Verification items for this drawing (mm, ordinates from the low corner). Coordinates: 2 decimals unless noted, no trailing zeros. Write each loop counter-clockwise with the first axis right and the second up, starting at its lowest first coordinate (ties: lowest second). Pieces come first, ordered by that corner, then holes.
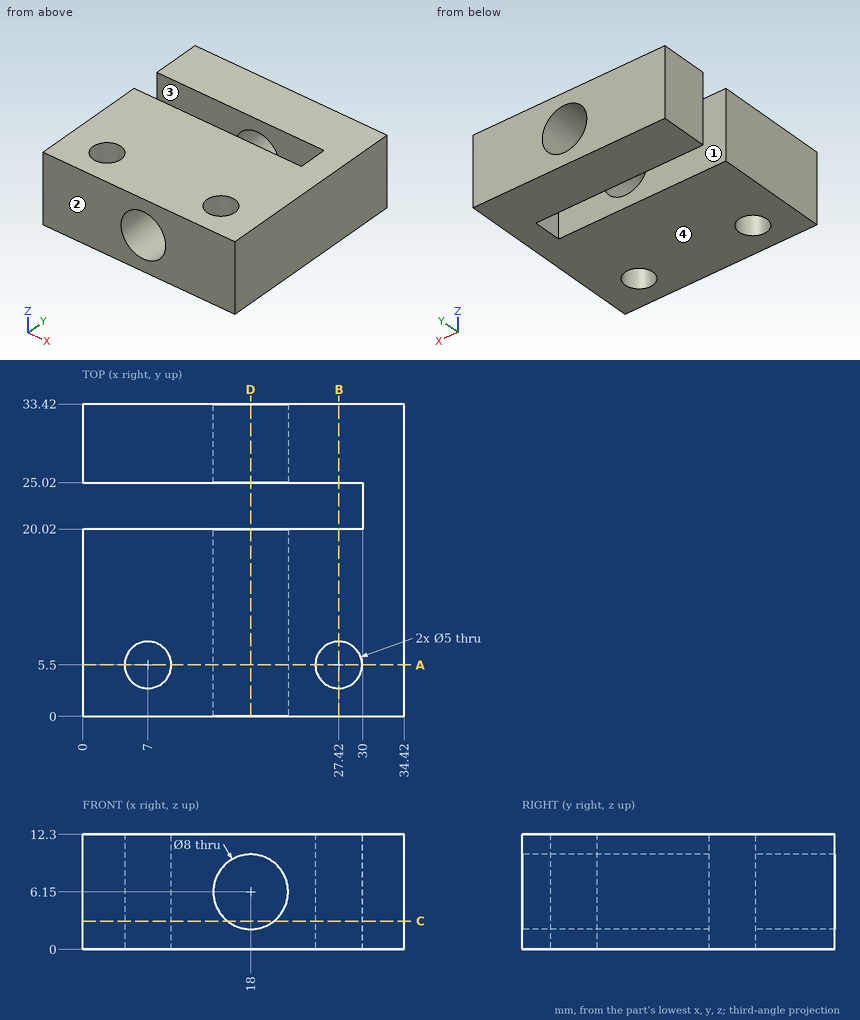
1. Sectioned sample at D-D, the plane x = 18. Record the boundary of the cut face in (y, z).
Computed values:
outline: (0, 0) - (20.02, 0) - (20.02, 2.15) - (0, 2.15) - close; (0, 10.15) - (20.02, 10.15) - (20.02, 12.3) - (0, 12.3) - close; (25.02, 0) - (33.42, 0) - (33.42, 2.15) - (25.02, 2.15) - close; (25.02, 10.15) - (33.42, 10.15) - (33.42, 12.3) - (25.02, 12.3) - close
2. Thickness scan on line 1 along Y through (x, z) = (27.42, 3.75); line 2 along X through (y, z) = (14, 6.15); line 3 along Y through (x, z) = (10.5, 7). Record the ranges inside material, lowest first.
Computed values:
line 1: y = 0 to 3, 8 to 20.02, 25.02 to 33.42
line 2: x = 0 to 14, 22 to 34.42
line 3: y = 0 to 20.02, 25.02 to 33.42
3. Sectioned sample at A-A, the plane y = 5.5. Record the boundary of the cut face in (x, z), and give its area (3 significant figures).
Computed values:
outline: (0, 0) - (4.5, 0) - (4.5, 12.3) - (0, 12.3) - close; (9.5, 0) - (24.92, 0) - (24.92, 12.3) - (9.5, 12.3) - close; (29.92, 0) - (34.42, 0) - (34.42, 12.3) - (29.92, 12.3) - close; hole circle Ø8 at (18, 6.15)
area: 250 mm2
4. Sectioned sample at C-C, the plane z = 3. Record the boundary of the cut face in (x, y), and give its area (3 significant figures).
Computed values:
outline: (0, 0) - (15.53, 0) - (15.53, 20.02) - (0, 20.02) - close; (0, 25.02) - (15.53, 25.02) - (15.53, 33.42) - (0, 33.42) - close; (20.47, 0) - (34.42, 0) - (34.42, 33.42) - (20.47, 33.42) - (20.47, 25.02) - (30, 25.02) - (30, 20.02) - (20.47, 20.02) - close; hole circle Ø5 at (7, 5.5); hole circle Ø5 at (27.42, 5.5)
area: 821 mm2
5. Gauge pin test, flat ends, axial feed: pin 1 Ø5 at (y, z) = (9, 7.5) entering from -X; pin 2 Ø5 at (x, z) = (18, 6.15) entering from +Y. Record the tip position at first contact, or that the pin passes through.
Computed values:
pin 1: stops at x = 0
pin 2: passes through
6. Draft check along Y on the marked faces 1, 2, 3 and 4. Enter one of: released by +Y, released by -Y, zero draft, split by the parting line, or undercut.
Computed values:
face 1: undercut
face 2: released by -Y
face 3: undercut
face 4: zero draft
7. Sectioned sample at B-B, the plane x = 27.42. Record the boundary of the cut face in (y, z).
Computed values:
outline: (0, 0) - (3, 0) - (3, 12.3) - (0, 12.3) - close; (8, 0) - (20.02, 0) - (20.02, 12.3) - (8, 12.3) - close; (25.02, 0) - (33.42, 0) - (33.42, 12.3) - (25.02, 12.3) - close
